from build123d import *

# Parameters (mm, degrees)
SKETCH1_W           = 76.2
SKETCH1_H           = 6.35
BOSS_EXTRUDE1_DEPTH = 558.8
SKETCH2_W           = 12.7
SKETCH2_H           = 6.35
CUT_EXTRUDE1_DEPTH  = 561.133352426
SKETCH3_W           = 50.8
SKETCH3_H           = 6.35
BOSS_EXTRUDE2_DEPTH = 6.35


with BuildPart() as part:
    # Sketch1 → Boss-Extrude1 (new body)
    with BuildSketch(Plane.XY):
        with Locations((0, 41.275)):
            Rectangle(SKETCH1_W, SKETCH1_H)
    extrude(amount=BOSS_EXTRUDE1_DEPTH)

    # Sketch2 → Cut-Extrude1 (cut, through all)
    with BuildSketch(Plane(origin=(0, 44.45, 0), x_dir=(1, 0, 0), z_dir=(0, 1, 0))):
        with Locations((12.7, -279.4)):
            Rectangle(SKETCH2_W, SKETCH2_H)
        with Locations((-12.7, -279.4)):
            Rectangle(SKETCH2_W, SKETCH2_H)
    extrude(amount=-CUT_EXTRUDE1_DEPTH, mode=Mode.SUBTRACT)

    # Sketch3 → Boss-Extrude2 (add)
    with BuildSketch(Plane(origin=(38.1, 0, 0), x_dir=(0, 0, -1), z_dir=(1, 0, 0))):
        with Locations((-381, 41.275)):
            Rectangle(SKETCH3_W, SKETCH3_H)
        with Locations((-279.4, 41.275)):
            Rectangle(SKETCH3_W, SKETCH3_H)
        with Locations((-177.8, 41.275)):
            Rectangle(SKETCH3_W, SKETCH3_H)
        with Locations((-76.2, 41.275)):
            Rectangle(SKETCH3_W, SKETCH3_H)
    extrude(amount=BOSS_EXTRUDE2_DEPTH)


solid = part.part
Can you work these out from the model? Positions are in its coordinate system, mm. Coordinates: 2 decimals unless noted, no trailing zeros. Loops run counter-clockwise (first coordinate to the right, second up) from the corner with the lowest first, then second, coordinate; pieces in that order, holes last. Notation, with made-up numbers: M 23,40 L 78,40 A12 cw 78,51 Z; hole C -4.5,82.5 d11. An arc over 180 degrees is marked long. Answer as CSV lines item,"result". Start each with the question number.
1. Suppose I cut it at B-B, the plane z = 518. List the corners of the cut face in (x, y) for me.
2. Suppose I cut it at A-A, the plane y = 39.5. List the corners of the cut face in (x, z) for me (3 decimals).
3. For pin 1 Ø1.9 at (x, y) = (40.5, 42) entering from +Z; pin 2 Ø3 at (x, y) = (42.5, 40.5) entering from -Z; pin 3 Ø1.9 at (y, z) = (42.5, 507) entering from +X, each with a flat end and sliding along its axis, tell me the tip position at first contact or that it passes through.
4. If I drill on probe 1 along Z at (x, y) = (41.5, 40); probe 2 along Z at (x, y) = (-10, 39.25) (3 decimals); probe 3 along X at (y, z) = (41, 327.5), over which ranges is the centre line in solid material (lowest first)? Write a range as [from, to].
Output:
1,outline,"M -38.1,38.1 L 38.1,38.1 L 38.1,44.45 L -38.1,44.45 Z"
2,outline,"M -38.1,0 L 38.1,0 L 38.1,50.8 L 44.45,50.8 L 44.45,101.6 L 38.1,101.6 L 38.1,152.4 L 44.45,152.4 L 44.45,203.2 L 38.1,203.2 L 38.1,254 L 44.45,254 L 44.45,304.8 L 38.1,304.8 L 38.1,355.6 L 44.45,355.6 L 44.45,406.4 L 38.1,406.4 L 38.1,558.8 L -38.1,558.8 Z; hole M -19.05,276.225 L -6.35,276.225 L -6.35,282.575 L -19.05,282.575 Z; hole M 6.35,276.225 L 19.05,276.225 L 19.05,282.575 L 6.35,282.575 Z"
3,pin 1,"stops at z = 406.4"
3,pin 2,"stops at z = 50.8"
3,pin 3,"stops at x = 38.1"
4,probe 1,"z = [50.8, 101.6], [152.4, 203.2], [254, 304.8], [355.6, 406.4]"
4,probe 2,"z = [0, 276.225], [282.575, 558.8]"
4,probe 3,"x = [-38.1, 38.1]"
